```python
from build123d import *

# Parameters (mm, degrees)
F0_R     = 11.2522
F1_DEPTH = 4.064
F2_COUNT = 2


with BuildPart() as f1:
    # F0 (on Top) → F1 (new body)
    with BuildSketch(Plane.XY):
        with BuildLine():
            ThreePointArc((-15.669299, 0), (0, -15.669299), (15.669299, 0))
            ThreePointArc((15.669299, 0), (0, 15.669299), (-15.669299, 0))
        make_face()
        Circle(F0_R, mode=Mode.SUBTRACT)
        with BuildLine():
            Line((15.669299, -34.433249), (15.669299, 0))
            ThreePointArc((15.669299, 0), (0, -15.669299), (-15.669299, 0))
            Line((-15.669299, 0), (-15.669299, -34.433249))
            Line((-15.669299, -34.433249), (-4.313127, -44.288438))
            Line((-4.313127, -44.288438), (6.474976, -44.288438))
            Line((6.474976, -44.288438), (15.669299, -34.433249))
        make_face()
    extrude(amount=F1_DEPTH)

    # F2: F1 ×2 about axis
    f2_axis = Axis((0, 0, 4.064), (0, 0, 1))


with BuildPart() as f1_1:
    add(f1.part)
    for i in range(1, F2_COUNT):
        add(f1.part.rotate(f2_axis, i * 360 / F2_COUNT))


solid = f1_1.part
```
Geometry check sheet. Reference: the model listing, model coordinates, mm. Give positions to 0.01 mm unless a question says otherwise; leave off trailing zeros. Loops run counter-clockwise (first coordinate to the right, second up) from the corner with the lowest first, then second, coordinate; pieces in that order, holes last. Notation, with made-up numbers: M 20.5,86.25 L 54.5,86.25 A15 ccw 54.5,113.25 Z; hole C 76.5,-25 d4. An arc over 180 degrees is marked long. Write item = value, one per line.
(1) Sectioned sample at A-A, the plane y = 0. Record the cut outline in (x, z).
Answer below:
outline = M -15.67,0 L -11.25,0 L -11.25,4.06 L -15.67,4.06 Z; M 11.25,0 L 15.67,0 L 15.67,4.06 L 11.25,4.06 Z
(2) Gauge pin test, flat end, axial feed: pin 1 Ø10 at (x, y) = (1.5, -1) entering from -Z. Record the tip position at first contact, or that the pin passes through.
Answer below:
pin_1 = through
(3) Material ranges on line 1 (Y direction, x = 0, z = 2.4); line 2 (Y direction, x = 7, z = 3.05); line 3 (X direction, y = -9, z = 1.25), recorded low to high. Write a range as [from, to].
Answer below:
line_1 = [-44.29, -11.25], [11.25, 44.29]
line_2 = [-43.73, -8.81], [8.81, 41.96]
line_3 = [-15.67, -6.75], [6.75, 15.67]
(4) Sectioned sample at C-C, the plane x = 0. Record the cut outline in (y, z), plus the area to 3 significant figures.
Answer below:
outline = M -44.29,0 L -11.25,0 L -11.25,4.06 L -44.29,4.06 Z; M 11.25,0 L 44.29,0 L 44.29,4.06 L 11.25,4.06 Z
area = 269 mm2
(5) Release check for a two-part mould opening along X. For faces 1 (the face through (-1.465, 11.156, 2.004)), 2 (the face through (-15.669, 0, 2)), 3 (the face through (15.669, 0, 2)) record: released by +X, released by -X, zero draft, split by the parting line, or undercut.
Answer below:
face_1 = undercut
face_2 = released by -X
face_3 = released by +X
(6) Sectioned sample at B-B, the plane z = 3.45. Record the cut outline in (x, y), plus the area to 3 significant figures.
Answer below:
outline = M -15.67,-34.43 L -4.31,-44.29 L 6.47,-44.29 L 15.67,-34.43 L 15.67,34.43 L 4.31,44.29 L -6.47,44.29 L -15.67,34.43 Z; hole C 0,0 d22.5
area = 2,180 mm2
